Can you work these out from the model? Positions are in its coordinate system, mm. Face numbers are marked on the shaded views. A direction names the side the tool comes from. Give positions to 0.01 mm unless a question says otherwise; leave off trailing zeros. Loops run counter-clockwise (first coordinate to the right, second up) from the corner with the lowest first, then second, coordinate; pieces in that order, holes last. Notation, with made-up numbers: M 41,-24 L 45,-24 A32 cw 45,15 Z; hole C 82,39.5 d2. An arc over 180 degrees is marked long. Use CSV: the item, a comma, the result in double quotes.
Autodesk Inventor part; units mm, degrees
ref_plane "YZ Plane" through (0, 0, 0) normal (1, 0, 0) x (0, 1, 0)
ref_plane "XZ Plane" through (0, 0, 0) normal (0, 1, 0) x (-1, 0, 0)
ref_plane "XY Plane" through (0, 0, 0) normal (0, 0, 1) x (1, 0, 0)
sketch "Sketch3" plane through (0, 0, 0) normal (0, 0, 1) x (1, 0, 0)
  circle A0 centre (0, 0) radius 25
  circle A1 centre (0, 0) radius 8.5
  dimension "d8" = 50
  dimension "d16" = 17
extrude "Extrusion3" add sketch "Sketch3" along normal blind 10 contours A0 | A1
sketch "Sketch4" plane through (0, 0, 10) normal (0, 0, 1) x (1, 0, 0)
  circle A0 centre (0, 0) radius 12
  circle A1 centre (0, 0) radius 8.5
  dimension "d12" = 24
  dimension "d17" = 17
extrude "Extrusion4" add sketch "Sketch4" along normal blind 8 contours A0 | A1
sketch "Sketch5" plane through (0, 0, 10) normal (0, 0, 1) x (1, 0, 0)
  point P0 (0, 0)
sketch "Sketch6" plane through (0, 0, 18) normal (0, 0, 1) x (1, 0, 0)
  circle A0 centre (0, 0) radius 8.5
  dimension "d18" = 17
extrude "Extrusion5" cut sketch "Sketch6" against normal blind 30
sketch "Sketch7" plane through (0, 0, 18) normal (0, 0, 1) x (1, 0, 0)
  circle A0 centre (0, 0) radius 12
  line L0 (6.3883, 10.1583) -> (-6.3883, 10.1583)
  arc A1 (6.3883, 10.1583) -> (-6.3883, 10.1583) centre (0, 0) ccw
  arc A2 (6.3883, 10.1583) -> (-6.3883, 10.1583) centre (0, 0) ccw
extrude "Extrusion6" cut sketch "Sketch7" against normal blind 8 contours L0 A0 picked at (-1.322, 10.5474)
sketch "Sketch8" plane through (-6.3883, 10.1583, 18) normal (0, 1, 0) x (1, 0, 0)
  point P0 (6.3883, 18)
  point P1 (6.3883, 4)
hole "Hole1" at (0, 10.1583, 14) direction (0, -1, 0) diameter 6 end through all
properties part number "Project_Stationary_Wheel[1]"
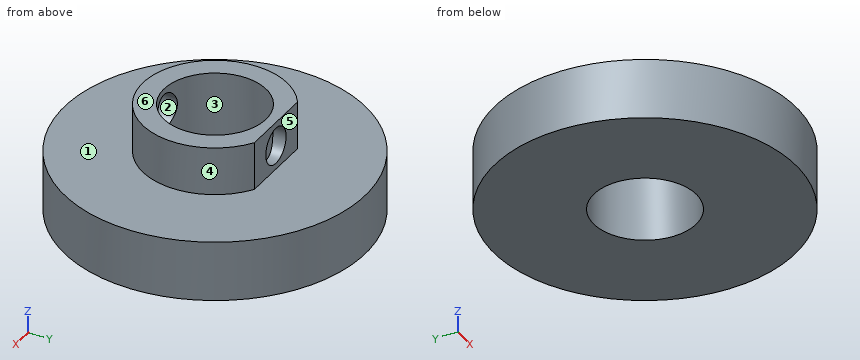
Q1. Please list where these lines run through material, in increasing order: L1, parallel to Y at x = 0, z = 8.5; L2, parallel to Z at x = 0, y = -10.35; L3, parallel to Y at x = 0, z = 10.75. Write a range as from..to.
Model answer:
L1,"-25..-8.5, 8.5..25"
L2,"0..11, 17..18"
L3,"-12..-8.5, 8.5..10.16"
Q2. If we mould it in two halves opening along Y, with no side actions, what happens to the marked faces 3, 4, 5 and 6? For each: released by +Y, released by -Y, zero draft, split by the parting line, or undercut.
Model answer:
face 3,"undercut"
face 4,"split by the parting line"
face 5,"released by +Y"
face 6,"zero draft"
Q3. I want a section at B-B, the plane y = 0. Please give me the cut outline in (x, z), then the cut area to 3 significant figures.
Model answer:
outline,"M -25,0 L -8.5,0 L -8.5,18 L -12,18 L -12,10 L -25,10 Z; M 8.5,0 L 25,0 L 25,10 L 12,10 L 12,18 L 8.5,18 Z"
area,"386 mm2"
Q4. For the marked faces 1 and 2, which set-ups out of +Z, -Z, +X, -X, +Y, -Y let a thin tool reach every point of the face, with its end or its side?
Model answer:
face 1,"+Z"
face 2,"+Y, -Y"
Q5. I want a section at C-C, the plane z = 14. Please give me the cut outline in (x, y), then the cut area to 3 significant figures.
Model answer:
outline,"M -6.39,10.16 A12 ccw -3,-11.62 L -3,-7.95 A8.5 cw -3,7.95 L -3,10.16 Z; M 3,-11.62 A12 ccw 6.39,10.16 L 3,10.16 L 3,7.95 A8.5 cw 3,-7.95 Z"
area,"177 mm2"
Q6. I want a section at D-D, the plane z = 1.5. Please give me the cut outline in (x, y), then the cut area to 3 significant figures.
Model answer:
outline,"C 0,0 d50; hole C 0,0 d17"
area,"1,740 mm2"
Q7. I'm going to push flat-ended pins straight in: P1, Ø2, axis at x = -7.5, z = 7, coming from the +Y side; P2, Ø1, axis at y = 5, z = 7, coming from the -X side; P3, Ø4, axis at x = -2.5, z = 13.5, coming from the +Y side; P4, Ø3.5, axis at x = 0, z = 14, coming from the -Y side. Where does each tip first touch, or does it pass through?
Model answer:
P1,"y = 24.14"
P2,"x = -24.59"
P3,"y = 10.16"
P4,"through"
Q8. I want a section at A-A, the plane x = 0. Please give me the cut outline in (y, z), then the cut area to 3 significant figures.
Model answer:
outline,"M -25,0 L -8.5,0 L -8.5,11 L -12,11 L -12,10 L -25,10 Z; M -12,17 L -8.5,17 L -8.5,18 L -12,18 Z; M 8.5,0 L 25,0 L 25,10 L 10.16,10 L 10.16,11 L 8.5,11 Z; M 8.5,17 L 10.16,17 L 10.16,18 L 8.5,18 Z"
area,"340 mm2"
